Verification items for the finished model (mm, model axes). Round coordinates to 2 decimals unless told otherwise and drop trailing zeros. Use CSV: the item, a comma, the result in double quotes.
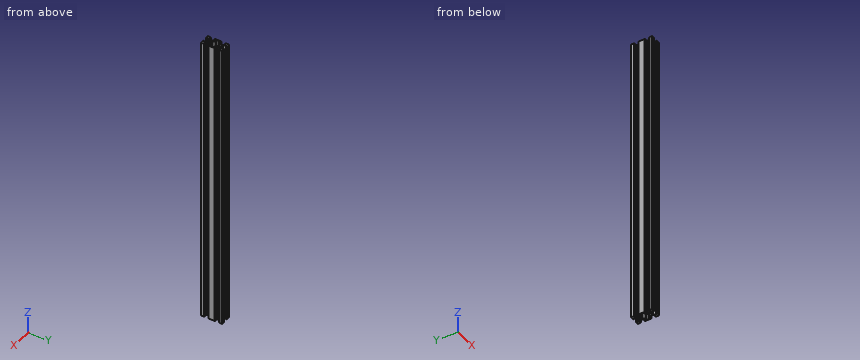
```python
from build123d import *

# Parameters (mm, degrees)
SKETCH_1_R      = 2.55
EXTRUDE_1_DEPTH = 550


with BuildPart() as part:
    # Эскиз1 → Бобышка-Вытянуть1 (new body)
    with BuildSketch(Plane.XY.offset(792.9)):
        Polygon((-8.2, -3.125), (-8.506400721, -3.125), (-10, -4.58), (-10, -15.42), (-8.506400721, -16.875), (-8.2, -16.875), (-8.2, -14.5), (-7.00202244, -14.5), (-3.9, -17.521856474), (-3.9, -19.8), (-3.7, -20), (-3.9, -20.2), (-3.9, -22.478143526), (-7.00202244, -25.5), (-8.2, -25.5), (-8.2, -23.125), (-8.506400721, -23.125), (-10, -24.58), (-10, -30), (-4.58, -30), (-3.125, -28.506400721), (-3.125, -28.2), (-5.5, -28.2), (-5.5, -27.00202244), (-2.478143526, -23.9), (-0.2, -23.9), (0, -23.7), (0.2, -23.9), (2.478143526, -23.9), (5.5, -27.00202244), (5.5, -28.2), (3.125, -28.2), (3.125, -28.506400721), (4.58, -30), (10, -30), (10, -24.58), (8.506400721, -23.125), (8.2, -23.125), (8.2, -25.5), (7.00202244, -25.5), (3.9, -22.478143526), (3.9, -20.2), (3.7, -20), (3.9, -19.8), (3.9, -17.521856474), (7.00202244, -14.5), (8.2, -14.5), (8.2, -16.875), (8.506400721, -16.875), (10, -15.42), (10, -4.58), (8.506400721, -3.125), (8.2, -3.125), (8.2, -5.5), (7.00202244, -5.5), (3.9, -2.478143526), (3.9, -0.2), (3.7, 0), (3.9, 0.2), (3.9, 2.478143526), (7.00202244, 5.5), (8.2, 5.5), (8.2, 3.125), (8.506400721, 3.125), (10, 4.58), (10, 10), (4.58, 10), (3.125, 8.506400721), (3.125, 8.2), (5.5, 8.2), (5.5, 7.00202244), (2.478143526, 3.9), (0.2, 3.9), (0, 3.7), (-0.2, 3.9), (-2.478143526, 3.9), (-5.5, 7.00202244), (-5.5, 8.2), (-3.125, 8.2), (-3.125, 8.506400721), (-4.58, 10), (-10, 10), (-10, 4.58), (-8.506400721, 3.125), (-8.2, 3.125), (-8.2, 5.5), (-7.00202244, 5.5), (-3.9, 2.478143526), (-3.9, 0.2), (-3.7, 0), (-3.9, -0.2), (-3.9, -2.478143526), (-7.00202244, -5.5), (-8.2, -5.5), align=None)
        Circle(SKETCH_1_R, mode=Mode.SUBTRACT)
        with Locations((0, -20)):
            Circle(SKETCH_1_R, mode=Mode.SUBTRACT)
        Polygon((-2.478143526, -3.9), (2.478143526, -3.9), (5.5, -7.00202244), (8.2, -7.00202244), (8.2, -12.99797756), (5.5, -12.99797756), (2.478143526, -16.1), (-2.478143526, -16.1), (-5.5, -12.99797756), (-8.2, -12.99797756), (-8.2, -7.00202244), (-5.5, -7.00202244), align=None, mode=Mode.SUBTRACT)
    extrude(amount=-EXTRUDE_1_DEPTH)


solid = part.part
```
Q1. Section check A-A (z = 439.5). State how many separate pieces and enclosed holes the cut face has, plus the area to 3 significant figures.
Filled in:
separate pieces,"1"
enclosed holes,"3"
area,"303 mm²"
Q2. Material ranges on L1, parallel to Y at x = 0, z = 433.5; L2, parallel to X at y = -20.5, z = 507.5; L3, parallel to X at y = 3.5, z = 509.5, recorded low to high.
Filled in:
L1,"-23.7 to -22.55, -17.45 to -16.1, -3.9 to -2.55, 2.55 to 3.7"
L2,"-3.9 to -2.5, 2.5 to 3.9"
L3,"-8.89 to -8.2, -4.95 to 4.95, 8.2 to 8.89"
Q3. Go/stop test with flat-tipped pins: P1, Ø2.5, axis at y = -21, z = 438.5, coming from the -X side; P2, Ø0.7, axis at y = -16, z = 429.5, coming from the -X side; P3, Ø3, axis at x = -3, z = 422.5, coming from the -Y side. Record where each tip stops, or that it passes through.
Filled in:
P1,"x = -3.9"
P2,"x = -9.76"
P3,"y = -29.92"
